Autodesk Inventor part; units mm, degrees
ref_plane "ip_st_1_1_XY" through (2, 4.5, 0) normal (1, 0, 0) x (0, 0, -1)
ref_plane "ip_st_1_1_YZ" through (2, 4.5, 0) normal (0, 0, -1) x (0, 1, 0)
ref_plane "ip_st_1_1_ZX" through (2, 4.5, 0) normal (0, 1, 0) x (1, 0, 0)
sketch "Sketch_2" plane through (0, 0, 0) normal (0, 0, 1) x (1, 0, 0)
  line L0 (4, 0) -> (0, 0)
  arc A0 (0, 3.15) -> (0.15, 3) centre (0.15, 3.15) ccw
  line L1 (0.15, 3) -> (3.85, 3)
  arc A1 (3.85, 3) -> (4, 3.15) centre (3.85, 3.15) ccw
  line L2 (4, 3.15) -> (4, 3.6)
  line L3 (4, 3.6) -> (3.75, 3.6)
  line L4 (3.75, 3.6) -> (3.75, 3.865)
  line L5 (3.75, 3.865) -> (2.6378, 3.865)
  arc A2 (1.3622, 3.865) -> (2.6378, 3.865) centre (2, 4.5) ccw
  line L6 (1.3622, 3.865) -> (0.25, 3.865)
  line L7 (0.25, 3.865) -> (0.25, 3.6)
  line L8 (0.25, 3.6) -> (0, 3.6)
  line L9 (0, 3.6) -> (0, 3.15)
revolve "Revolution1" add sketch "Sketch_2" angle 360 about axis through (4, 0, 0) along (1, 0, 0)
ref_plane "ip_st_1_1_XY" through (2, 4.5, 0) normal (1, 0, 0) x (0, 0, -1)
ref_plane "ip_st_1_1_YZ" through (2, 4.5, 0) normal (0, 0, -1) x (0, 1, 0)
ref_plane "ip_st_1_1_ZX" through (2, 4.5, 0) normal (0, 1, 0) x (1, 0, 0)
ref_plane "ip_st_1_10_XY" through (2, 0, -4.5) normal (1, 0, 0) x (0, 0, -1)
ref_plane "ip_st_1_10_YZ" through (2, 0, -4.5) normal (0, 0, -1) x (0, 1, 0)
ref_plane "ip_st_1_10_ZX" through (2, 0, -4.5) normal (0, 1, 0) x (1, 0, 0)
ref_plane "ip_st_1_11_XY" through (2, 2.25, -3.8971) normal (1, 0, 0) x (0, 0, -1)
ref_plane "ip_st_1_11_YZ" through (2, 2.25, -3.8971) normal (0, 0, -1) x (0, 1, 0)
ref_plane "ip_st_1_11_ZX" through (2, 2.25, -3.8971) normal (0, 1, 0) x (1, 0, 0)
ref_plane "ip_st_1_12_XY" through (2, 3.8971, -2.25) normal (1, 0, 0) x (0, 0, -1)
ref_plane "ip_st_1_12_YZ" through (2, 3.8971, -2.25) normal (0, 0, -1) x (0, 1, 0)
ref_plane "ip_st_1_12_ZX" through (2, 3.8971, -2.25) normal (0, 1, 0) x (1, 0, 0)
ref_plane "ip_st_1_2_XY" through (2, 3.8971, 2.25) normal (1, 0, 0) x (0, 0, -1)
ref_plane "ip_st_1_2_YZ" through (2, 3.8971, 2.25) normal (0, 0, -1) x (0, 1, 0)
ref_plane "ip_st_1_2_ZX" through (2, 3.8971, 2.25) normal (0, 1, 0) x (1, 0, 0)
ref_plane "ip_st_1_3_XY" through (2, 2.25, 3.8971) normal (1, 0, 0) x (0, 0, -1)
ref_plane "ip_st_1_3_YZ" through (2, 2.25, 3.8971) normal (0, 0, -1) x (0, 1, 0)
ref_plane "ip_st_1_3_ZX" through (2, 2.25, 3.8971) normal (0, 1, 0) x (1, 0, 0)
ref_plane "ip_st_1_4_XY" through (2, 0, 4.5) normal (1, 0, 0) x (0, 0, -1)
ref_plane "ip_st_1_4_YZ" through (2, 0, 4.5) normal (0, 0, -1) x (0, 1, 0)
ref_plane "ip_st_1_4_ZX" through (2, 0, 4.5) normal (0, 1, 0) x (1, 0, 0)
ref_plane "ip_st_1_5_XY" through (2, -2.25, 3.8971) normal (1, 0, 0) x (0, 0, -1)
ref_plane "ip_st_1_5_YZ" through (2, -2.25, 3.8971) normal (0, 0, -1) x (0, 1, 0)
ref_plane "ip_st_1_5_ZX" through (2, -2.25, 3.8971) normal (0, 1, 0) x (1, 0, 0)
ref_plane "ip_st_1_6_XY" through (2, -3.8971, 2.25) normal (1, 0, 0) x (0, 0, -1)
ref_plane "ip_st_1_6_YZ" through (2, -3.8971, 2.25) normal (0, 0, -1) x (0, 1, 0)
ref_plane "ip_st_1_6_ZX" through (2, -3.8971, 2.25) normal (0, 1, 0) x (1, 0, 0)
ref_plane "ip_st_1_7_XY" through (2, -4.5, 0) normal (1, 0, 0) x (0, 0, -1)
ref_plane "ip_st_1_7_YZ" through (2, -4.5, 0) normal (0, 0, -1) x (0, 1, 0)
ref_plane "ip_st_1_7_ZX" through (2, -4.5, 0) normal (0, 1, 0) x (1, 0, 0)
ref_plane "ip_st_1_8_XY" through (2, -3.8971, -2.25) normal (1, 0, 0) x (0, 0, -1)
ref_plane "ip_st_1_8_YZ" through (2, -3.8971, -2.25) normal (0, 0, -1) x (0, 1, 0)
ref_plane "ip_st_1_8_ZX" through (2, -3.8971, -2.25) normal (0, 1, 0) x (1, 0, 0)
ref_plane "ip_st_1_9_XY" through (2, -2.25, -3.8971) normal (1, 0, 0) x (0, 0, -1)
ref_plane "ip_st_1_9_YZ" through (2, -2.25, -3.8971) normal (0, 0, -1) x (0, 1, 0)
ref_plane "ip_st_1_9_ZX" through (2, -2.25, -3.8971) normal (0, 1, 0) x (1, 0, 0)
ref_plane "ip_st_1a_XY" through (0, 0, 0) normal (1, 0, 0) x (0, 0, -1)
ref_plane "ip_st_1a_YZ" through (0, 0, 0) normal (0, 0, -1) x (0, 1, 0)
ref_plane "ip_st_1a_ZX" through (0, 0, 0) normal (0, 1, 0) x (1, 0, 0)
ref_plane "ip_st_2a_XY" through (0.25, 0, 0) normal (1, 0, 0) x (0, 0, -1)
ref_plane "ip_st_2a_YZ" through (0.25, 0, 0) normal (0, 0, -1) x (0, 1, 0)
ref_plane "ip_st_2a_ZX" through (0.25, 0, 0) normal (0, 1, 0) x (1, 0, 0)
properties part number "MF126ZZ Inner Ring"
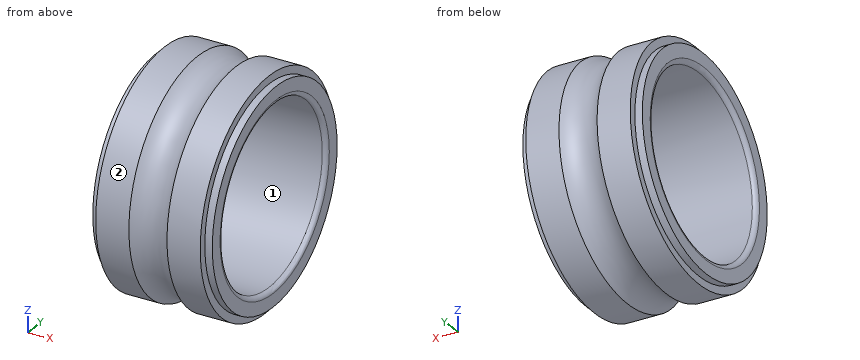
Read the model definition and answer for the solid it produces. Units are mm, in the model's axes. Face numbers are marked on the shaded views. Round coordinates to 2 decimals unless told otherwise and drop trailing zeros. Write each loop counter-clockwise with the first axis right and the second up, starting at its lowest first coordinate (ties: lowest second). Pieces come first, ordered by that corner, then holes. Notation, with made-up numbers: (48, -30.5) - (105, -30.5) arc R30 cw to (105, 2.5) - close; hole circle Ø3 at (83, 60.5). An arc over 180 degrees is marked (long way). Use CSV: the item, a comma, the result in double quotes.
Q1. Straight lines are drawn through the part: line 1 along Z through (x, y) = (2, 0); line 2 along Z through (x, y) = (1.25, 0) (3 decimals); line 3 along X through (y, z) = (0.75, 3.75). For each, find the intervals that lie inside material, in ascending order.
Values:
line 1,"z = -3.6 to -3, 3 to 3.6"
line 2,"z = -3.865 to -3, 3 to 3.865"
line 3,"x = 0.25 to 1.41, 2.59 to 3.75"
Q2. Each of these flat-tipped pins is pushed along its axis until it touches: pin 1 Ø3 at (y, z) = (-2.5, -1) entering from +X; pin 2 Ø1.5 at (x, z) = (1, -1.5) entering from +Y. Where does it stop, or does it pass through?
Values:
pin 1,"stops at x = 4"
pin 2,"stops at y = 3.79"
Q3. Find section D-D, the plane x = 2.35. Write down the section's boundary in (y, z), then the cut area to 3 significant figures.
Values:
outline,"circle Ø7.34 at (0, 0); hole circle Ø6 at (0, 0)"
area,"14.1 mm²"
Q4. Find section A-A, the plane z = 0. Write down the section's boundary in (x, y) (3 decimals), then the cut area to 3 significant figures.
Values:
outline,"(0, -3.6) - (0.25, -3.6) - (0.25, -3.865) - (1.362, -3.865) arc R0.9 cw to (2.638, -3.865) - (3.75, -3.865) - (3.75, -3.6) - (4, -3.6) - (4, -3.15) arc R0.15 ccw to (3.85, -3) - (0.15, -3) arc R0.15 ccw to (0, -3.15) - close; (0, 3.15) arc R0.15 ccw to (0.15, 3) - (3.85, 3) arc R0.15 ccw to (4, 3.15) - (4, 3.6) - (3.75, 3.6) - (3.75, 3.865) - (2.638, 3.865) arc R0.9 cw to (1.362, 3.865) - (0.25, 3.865) - (0.25, 3.6) - (0, 3.6) - close"
area,"6.17 mm²"
Q5. Find section C-C, the plane x = 3.1. Write down the section's boundary in (y, z) (3 decimals), then the cut area to 3 significant figures.
Values:
outline,"circle Ø7.73 at (0, 0); hole circle Ø6 at (0, 0)"
area,"18.7 mm²"
Q6. Determine the mould class of the marked faces 1 and 2 for opening direction Y: +Y half, -Y half, draft (parallel to the pull), parting line (faces both ways), or undercut.
Values:
face 1,"undercut"
face 2,"parting line"
